Input: part model. Units: mm. Frame: model coordinates. A direction names the side the tool comes from. Coordinates: 2 decimals unless noted, no trailing zeros. Order: outer loops, then holes, each group sorted by start corner. A loop starts at its lowest first (then second) coordinate and runs counter-clockwise, first axis right, second up. Notation, with made-up numbers: (68.5, 71.25) -> (120.5, 71.25) arc R6 ccw to (120.5, 77.25) -> close; hole circle Ø5 at (54, 86). An arc over 180 degrees is marked (long way). Answer as CSV lines item,"result".
from build123d import *

# Parameters (mm, degrees)
BOSS_EXTRUDE1_DEPTH      = 73.75
BOSS_EXTRUDE1_DEPTH_BACK = 73.75
SKETCH1_W                = 5
SKETCH1_H                = 116
SKETCH2_R                = 1.5
CUT_EXTRUDE1_DEPTH       = 139.275314138
CUT_EXTRUDE2_START       = -10
CUT_EXTRUDE2_OUTLINE_R   = 3.15
CUT_EXTRUDE2_OUTLINE_R_2 = 1.5
CUT_EXTRUDE2_DEPTH       = 7.525862169
SKETCH4_W                = 147.5
SKETCH4_H                = 21
CUT_EXTRUDE3_DEPTH       = 4
SKETCH6_R                = 1.65
CUT_EXTRUDE4_DEPTH       = 139.275314138
SKETCH7_R                = 3.15
CUT_EXTRUDE6_DEPTH       = 10
SKETCH8_W                = 30
SKETCH8_H                = 30
BOSS_EXTRUDE2_DEPTH      = 7
SKETCH9_W                = 34
SKETCH9_H                = 30
BOSS_EXTRUDE3_DEPTH      = 30
SKETCH10_W               = 34
SKETCH10_H               = 30
BOSS_EXTRUDE4_DEPTH      = 30


# Read off the part's stored shape, not the designer's step: Cut-Extrude2
with BuildPart() as part:
    # Sketch1 → Boss-Extrude1 (new, two sides: drawn at the far end of the back side and taken through both)
    with BuildSketch(Plane.XY.offset(-BOSS_EXTRUDE1_DEPTH_BACK)):
        Polygon((10, 0), (5, 0), (5, -116), (10, -116), (15, -87), (15, -58), (15, -29), align=None)
        with Locations((2.5, -58)):
            Rectangle(SKETCH1_W, SKETCH1_H)
    extrude(amount=BOSS_EXTRUDE1_DEPTH + BOSS_EXTRUDE1_DEPTH_BACK)

    # Sketch2 → Cut-Extrude1 (cut, through all)
    with BuildSketch(Plane(origin=(15, 0, 0), x_dir=(0, 0, -1), z_dir=(1, 0, 0))):
        with Locations(Location((60, -106, 0), (0, 0, 90))):
            Circle(SKETCH2_R)
        with Locations(Location((45, -106, 0), (0, 0, 90))):
            Circle(SKETCH2_R)
        with Locations(Location((22.5, -104.5, 0), (0, 0, 90))):
            Circle(SKETCH2_R)
        with Locations(Location((14.5, -104.5, 0), (0, 0, 90))):
            Circle(SKETCH2_R)
        with Locations(Location((-14.5, -104.5, 0), (0, 0, 90))):
            Circle(SKETCH2_R)
        with Locations(Location((-22.5, -104.5, 0), (0, 0, 90))):
            Circle(SKETCH2_R)
        with Locations(Location((-45, -106, 0), (0, 0, 90))):
            Circle(SKETCH2_R)
        with Locations(Location((-60, -106, 0), (0, 0, 90))):
            Circle(SKETCH2_R)
    extrude(amount=-CUT_EXTRUDE1_DEPTH, mode=Mode.SUBTRACT)

    # Cut-Extrude2 outline → Cut-Extrude2 (cut)
    # profile 1 of 8: a face of its own
    with BuildSketch(Plane(origin=(15, 0, 0), x_dir=(0, 0, -1), z_dir=(1, 0, 0)).offset(CUT_EXTRUDE2_START)):
        with Locations((60, -106)):
            Circle(CUT_EXTRUDE2_OUTLINE_R)
        with Locations((60, -106)):
            Circle(CUT_EXTRUDE2_OUTLINE_R_2, mode=Mode.SUBTRACT)
    # profile 2 of 8: a face of its own
    with BuildSketch(Plane(origin=(15, 0, 0), x_dir=(0, 0, -1), z_dir=(1, 0, 0)).offset(CUT_EXTRUDE2_START)):
        with Locations((22.5, -104.5)):
            Circle(CUT_EXTRUDE2_OUTLINE_R)
        with Locations((22.5, -104.5)):
            Circle(CUT_EXTRUDE2_OUTLINE_R_2, mode=Mode.SUBTRACT)
    # profile 3 of 8: a face of its own
    with BuildSketch(Plane(origin=(15, 0, 0), x_dir=(0, 0, -1), z_dir=(1, 0, 0)).offset(CUT_EXTRUDE2_START)):
        with Locations((45, -106)):
            Circle(CUT_EXTRUDE2_OUTLINE_R)
        with Locations((45, -106)):
            Circle(CUT_EXTRUDE2_OUTLINE_R_2, mode=Mode.SUBTRACT)
    # profile 4 of 8: a face of its own
    with BuildSketch(Plane(origin=(15, 0, 0), x_dir=(0, 0, -1), z_dir=(1, 0, 0)).offset(CUT_EXTRUDE2_START)):
        with Locations((14.5, -104.5)):
            Circle(CUT_EXTRUDE2_OUTLINE_R)
        with Locations((14.5, -104.5)):
            Circle(CUT_EXTRUDE2_OUTLINE_R_2, mode=Mode.SUBTRACT)
    # profile 5 of 8: a face of its own
    with BuildSketch(Plane(origin=(15, 0, 0), x_dir=(0, 0, -1), z_dir=(1, 0, 0)).offset(CUT_EXTRUDE2_START)):
        with Locations((-14.5, -104.5)):
            Circle(CUT_EXTRUDE2_OUTLINE_R)
        with Locations((-14.5, -104.5)):
            Circle(CUT_EXTRUDE2_OUTLINE_R_2, mode=Mode.SUBTRACT)
    # profile 6 of 8: a face of its own
    with BuildSketch(Plane(origin=(15, 0, 0), x_dir=(0, 0, -1), z_dir=(1, 0, 0)).offset(CUT_EXTRUDE2_START)):
        with Locations((-22.5, -104.5)):
            Circle(CUT_EXTRUDE2_OUTLINE_R)
        with Locations((-22.5, -104.5)):
            Circle(CUT_EXTRUDE2_OUTLINE_R_2, mode=Mode.SUBTRACT)
    # profile 7 of 8: a face of its own
    with BuildSketch(Plane(origin=(15, 0, 0), x_dir=(0, 0, -1), z_dir=(1, 0, 0)).offset(CUT_EXTRUDE2_START)):
        with Locations((-45, -106)):
            Circle(CUT_EXTRUDE2_OUTLINE_R)
        with Locations((-45, -106)):
            Circle(CUT_EXTRUDE2_OUTLINE_R_2, mode=Mode.SUBTRACT)
    # profile 8 of 8: a face of its own
    with BuildSketch(Plane(origin=(15, 0, 0), x_dir=(0, 0, -1), z_dir=(1, 0, 0)).offset(CUT_EXTRUDE2_START)):
        with Locations((-60, -106)):
            Circle(CUT_EXTRUDE2_OUTLINE_R)
        with Locations((-60, -106)):
            Circle(CUT_EXTRUDE2_OUTLINE_R_2, mode=Mode.SUBTRACT)
    extrude(amount=CUT_EXTRUDE2_DEPTH, mode=Mode.SUBTRACT)

    # Sketch4 → Cut-Extrude3 (cut)
    with BuildSketch(Plane.ZY):
        with Locations((0, -105.5)):
            Rectangle(SKETCH4_W, SKETCH4_H)
    extrude(amount=-CUT_EXTRUDE3_DEPTH, mode=Mode.SUBTRACT)

    # Sketch6 → Cut-Extrude4 (cut, through all)
    with BuildSketch(Plane(origin=(15, 0, 0), x_dir=(0, 0, -1), z_dir=(1, 0, 0))):
        with Locations(Location((12.25, -16, 0), (0, 0, 90))):
            Circle(SKETCH6_R)
        with Locations(Location((22.25, -16, 0), (0, 0, 90))):
            Circle(SKETCH6_R)
        with Locations(Location((-22.25, -16, 0), (0, 0, 270))):
            Circle(SKETCH6_R)
        with Locations(Location((-12.25, -16, 0), (0, 0, 270))):
            Circle(SKETCH6_R)
    extrude(amount=-CUT_EXTRUDE4_DEPTH, mode=Mode.SUBTRACT)

    # Sketch7 → Cut-Extrude6 (cut)
    with BuildSketch(Plane(origin=(15, 0, 0), x_dir=(0, 0, -1), z_dir=(1, 0, 0))):
        with Locations(Location((22.25, -16, 0), (0, 0, 90))):
            Circle(SKETCH7_R)
        with Locations(Location((12.25, -16, 0), (0, 0, 90))):
            Circle(SKETCH7_R)
        with Locations(Location((-12.25, -16, 0), (0, 0, 270))):
            Circle(SKETCH7_R)
        with Locations(Location((-22.25, -16, 0), (0, 0, 270))):
            Circle(SKETCH7_R)
    extrude(amount=-CUT_EXTRUDE6_DEPTH, mode=Mode.SUBTRACT)

    # Sketch8 → Boss-Extrude2 (add)
    with BuildSketch(Plane.ZY):
        with Locations((58.75, -15)):
            Rectangle(SKETCH8_W, SKETCH8_H)
        with Locations((-58.75, -15)):
            Rectangle(SKETCH8_W, SKETCH8_H)
    extrude(amount=BOSS_EXTRUDE2_DEPTH)

    # Sketch9 → Boss-Extrude3 (add)
    with BuildSketch(Plane.XY.offset(73.75)):
        with Locations((10, -15)):
            Rectangle(SKETCH9_W, SKETCH9_H)
    extrude(amount=-BOSS_EXTRUDE3_DEPTH)

    # Sketch10 → Boss-Extrude4 (add)
    with BuildSketch(Plane(origin=(0, 0, -73.75), x_dir=(-1, 0, 0), z_dir=(0, 0, -1))):
        with Locations((-10, -15)):
            Rectangle(SKETCH10_W, SKETCH10_H)
    extrude(amount=-BOSS_EXTRUDE4_DEPTH)


solid = part.part
1. Cut plane A-A (x = 22). Return the cut outline in (y, z).
Findings:
outline,"(-30, -73.75) -> (0, -73.75) -> (0, -43.75) -> (-30, -43.75) -> close; (-30, 43.75) -> (0, 43.75) -> (0, 73.75) -> (-30, 73.75) -> close"
2. Reachability of faces 1 (the face through (-3, -15, 43.75)), 2 (the face through (21, -30, 59)), 3 (the face through (9.21, -18.91, 23.46)) from +Z, -Z, +X, -X, +Y, -Y: full face, straight path, thin tool, end or side. Return the list, or none.
Findings:
face 1,"-X, +Y, -Y"
face 2,"+Z, -Z, +X, -Y"
face 3,"+X"
3. Ray query, line 1 along Z through (x, y) = (11, -16); line 2 along Y through (x, z) = (3, 12); line 3 along Y through (x, z) = (9, 45). Return the intervals inside material, ascending.
Findings:
line 1,"z = -73.75 to -25.4, -19.1 to -15.4, -9.1 to 9.1, 15.4 to 19.1, 25.4 to 73.75"
line 2,"y = -95 to -17.63, -14.37 to 0"
line 3,"y = -116 to -109.15, -102.85 to 0"
4. Cut plane C-C (y = -16). State how many separate pieces and enclosed holes the cut face has, plus the area to 3 significant figures.
Findings:
separate pieces,"5"
enclosed holes,"0"
area,"2,890 mm2"
5. Contact query for flat-ended pins moving along their axis: pin 1 (7 mm diameter, centred on y = -106, z = 60, fed in from +X); pin 2 (4 mm diameter, centred on y = -106, z = -60, fed in from +X); pin 3 (2 mm diameter, centred on x = -2, y = -77.5, fed in from +Z); pin 4 (2 mm diameter, centred on y = -25, z = -11.5, fed in from +X). Output: stop coordinate, or through.
Findings:
pin 1,"stops at x = 12.33"
pin 2,"stops at x = 5"
pin 3,"passes through"
pin 4,"stops at x = 14.48"
6. Cut plane B-B (z = 33). Return the cut outline in (x, y).
Findings:
outline,"(0, -95) -> (4, -95) -> (4, -116) -> (10, -116) -> (15, -87) -> (15, -29) -> (10, 0) -> (0, 0) -> close"
7. Cut plane D-D (y = -99). Return the cut outline in (x, z).
Findings:
outline,"(4, -73.75) -> (12.93, -73.75) -> (12.93, 73.75) -> (4, 73.75) -> close"
8. Mould query, pull axis Z, two halves, no side actions, for faces 4 (the face through (9.209, -19.005, 11.304)), 5 (the face through (0, -59, -1)), 6 (the face through (4, -105, -1)). Classes: released by +Z, released by -Z, zero draft, split by the parting line, or undercut.
Findings:
face 4,"undercut"
face 5,"undercut"
face 6,"zero draft"
